Source: CAD feature listing. Evaluate the final solid. Frame: model axes, mm. A direction names the side the tool comes from. Give positions to 0.01 mm unless a question says otherwise; leave off trailing zeros. Order: outer loops, then holes, each group sorted by start corner. A loop starts at its lowest first (then second) coordinate and runs counter-clockwise, first axis right, second up.
1) Section A-A, the plane x = 0. Return loops of the section in (y, z), plus the area to 3 significant figures.
2) First-contact query: P1, Ø3.5, axis at x = -3, y = 3.5, coming from the -Z side; P2, Ø1, axis at y = 3, z = 2.5, coming from the +X side; P3, Ø3.5, axis at x = -4.5, y = 1.5, coming from the +Z side. Flat tips, straight axial feed; report the tip coordinate or a pass-through.
3) Draft query along Y for faces 4 (the face through (3, -0.05, 1)), 5 (the face through (-3.612, -0.532, 0.802)), 6 (the face through (-4.149, 3.838, 0.042)), 7 (the face through (3, -1, 0)). Return one class per face: released by +Y, released by -Y, zero draft, split by the parting line, or undercut.
4) Access query for faces 1 (the face through (2.48, 1.49, -0.33)), 2 (the face through (2.18, 4.53, -0.29)), 3 (the face through (-5.718, 2.599, -0.042)). Directions: +Z, -Z, +X, -X, +Y, -Y. A direction counts if a zero-diameter tool reaches every point of the face in a straight line with its end or side. Return the directions, or none.
5) Section B-B, the plane z = 0. Return loops of the section in (x, y), plus the area to 3 significant figures.
6) Section C-C, the plane y = 3.5. Return loops of the section in (x, z).
7) Material intervals for line 1 (Y direction, x = -3.47, z = -0.75); line 2 (X direction, y = 0.1, z = 0); line 3 (Y direction, x = -3, z = -2), sorted ascending.
8) Section D-D, the plane x = -3.47. Return loops of the section in (y, z), plus the area to 3 significant figures.
```python
from build123d import *

# Parameters (mm, degrees)
SKETCH1_R                = 3
SKETCH1_R_2              = 2.5
BOSS_EXTRUDE1_DEPTH      = 5
BOSS_EXTRUDE1_DEPTH_BACK = 1
SKETCH2_R                = 2.25
SKETCH2_R_2              = 1.5
BOSS_EXTRUDE2_DEPTH      = 3
BOSS_EXTRUDE2_DEPTH_BACK = 3
SKETCH3_R                = 1.5
CUT_EXTRUDE1_DEPTH       = 10.680826584
SKETCH4_R                = 2.5
CUT_EXTRUDE2_DEPTH       = 9.815804089
SKETCH5_R                = 0.566074209
SKETCH5_R_2              = 0.324906468
BOSS_EXTRUDE3_DEPTH      = 0.5
BOSS_EXTRUDE3_DEPTH_BACK = 0.5
SKETCH6_R                = 3.7
SKETCH6_R_2              = 3
BOSS_EXTRUDE4_DEPTH      = 0.95
SKETCH7_R                = 2.5
SKETCH7_R_2              = 2.2
BOSS_EXTRUDE5_DEPTH      = 0.95


with BuildPart() as part:
    # Sketch1 → Boss-Extrude1 (new, two sides)
    with BuildSketch(Plane(origin=(0, 0, 0), x_dir=(1, 0, 0), z_dir=(0, 1, 0))) as boss_extrude1_sk:
        with Locations(Location((0, 0, 0), (0, 0, 270))):
            Circle(SKETCH1_R)
        with Locations(Location((0, 0, 0), (0, 0, 270))):
            Circle(SKETCH1_R_2, mode=Mode.SUBTRACT)
    extrude(amount=BOSS_EXTRUDE1_DEPTH)
    extrude(boss_extrude1_sk.sketch, amount=-BOSS_EXTRUDE1_DEPTH_BACK)

    # Sketch2 → Boss-Extrude2 (add, two sides)
    with BuildSketch(Plane.XY) as boss_extrude2_sk:
        with Locations((-3.47, 2.5)):
            Circle(SKETCH2_R)
        with Locations((-3.47, 2.5)):
            Circle(SKETCH2_R_2, mode=Mode.SUBTRACT)
    extrude(amount=BOSS_EXTRUDE2_DEPTH)
    extrude(boss_extrude2_sk.sketch, amount=-BOSS_EXTRUDE2_DEPTH_BACK)

    # Sketch3 → Cut-Extrude1 (cut, through all)
    with BuildSketch(Plane.XY.offset(3)):
        with Locations((-3.47, 2.5)):
            Circle(SKETCH3_R)
    extrude(amount=-CUT_EXTRUDE1_DEPTH, mode=Mode.SUBTRACT)

    # Sketch4 → Cut-Extrude2 (cut, through all)
    with BuildSketch(Plane(origin=(0, 5, 0), x_dir=(1, 0, 0), z_dir=(0, 1, 0))):
        with Locations(Location((0, 0, 0), (0, 0, 270))):
            Circle(SKETCH4_R)
    extrude(amount=-CUT_EXTRUDE2_DEPTH, mode=Mode.SUBTRACT)

    # Sketch5 → Boss-Extrude3 (add, two sides)
    with BuildSketch(Plane.XY) as boss_extrude3_sk:
        with Locations((-3.318977868, 5.08019985)):
            Circle(SKETCH5_R)
        with Locations((-3.318977868, 5.08019985)):
            Circle(SKETCH5_R_2, mode=Mode.SUBTRACT)
    extrude(amount=BOSS_EXTRUDE3_DEPTH)
    extrude(boss_extrude3_sk.sketch, amount=-BOSS_EXTRUDE3_DEPTH_BACK)

    # Sketch6 → Boss-Extrude4 (add)
    with BuildSketch(Plane.XZ.offset(1)):
        with Locations(Location((0, 0, 0), (0, 0, 270))):
            Circle(SKETCH6_R)
        with Locations(Location((0, 0, 0), (0, 0, 170.405931773))):
            Circle(SKETCH6_R_2, mode=Mode.SUBTRACT)
    extrude(amount=-BOSS_EXTRUDE4_DEPTH)

    # Sketch7 → Boss-Extrude5 (add)
    with BuildSketch(Plane(origin=(0, 5, 0), x_dir=(1, 0, 0), z_dir=(0, 1, 0))):
        with Locations(Location((0, 0, 0), (0, 0, 270))):
            Circle(SKETCH7_R)
        with Locations(Location((0, 0, 0), (0, 0, 270))):
            Circle(SKETCH7_R_2, mode=Mode.SUBTRACT)
    extrude(amount=-BOSS_EXTRUDE5_DEPTH)


solid = part.part
```
From the geometry:
1. outline: (-1, -3.7) - (-0.05, -3.7) - (-0.05, -3) - (5, -3) - (5, -2.2) - (4.05, -2.2) - (4.05, -2.5) - (-1, -2.5) - close; (-1, 2.5) - (4.05, 2.5) - (4.05, 2.2) - (5, 2.2) - (5, 3) - (-0.05, 3) - (-0.05, 3.7) - (-1, 3.7) - close
1. area: 7.90 mm2
2. P1: stops at z = -3
2. P2: stops at x = 2.24
2. P3: stops at z = 3
3. face 4: undercut
3. face 5: zero draft
3. face 6: undercut
3. face 7: released by -Y
4. face 1: -Y
4. face 2: +Y, -Y
4. face 3: none
5. outline: (-3.76, 4.73) arc R2.25 ccw (long way) to (-3, 0.3) - (-3, -0.05) - (-3.7, -0.05) - (-3.7, -1) - (-2.5, -1) - (-2.5, 1.36) arc R1.5 cw (long way) to (-2.5, 3.64) - (-2.5, 4.05) - (-2.2, 4.05) - (-2.2, 5) - (-2.76, 5) arc R0.57 ccw (long way) to start; (2.2, 4.05) - (2.5, 4.05) - (2.5, -1) - (3.7, -1) - (3.7, -0.05) - (3, -0.05) - (3, 5) - (2.2, 5) - close; hole circle Ø0.65 at (-3.32, 5.08)
5. area: 12.2 mm2
6. outline: (-5.49, -3) - (-4.59, -3) - (-4.59, 3) - (-5.49, 3) - close; (-2.35, -3) - (-1.45, -3) - (-1.45, -2.62) arc R3 ccw (long way) to (-1.45, 2.62) - (-1.45, 3) - (-2.35, 3) - (-2.35, 0.85) arc R2.5 cw (long way) to (-2.35, -0.85) - close
7. line 1: y = -1 to -0.05, 0.25 to 1, 4 to 4.75
7. line 2: x = -3 to -2.5, 2.5 to 3
7. line 3: y = -1 to -0.05, 0.3 to 1.08, 3.92 to 4.7
8. outline: (-1, -1.28) - (-0.05, -1.28) - (-0.05, 1.28) - (-1, 1.28) - close; (0.25, -3) - (1, -3) - (1, 3) - (0.25, 3) - close; (4, -3) - (4.75, -3) - (4.75, -0.5) - (4.79, -0.5) - (4.79, 0.5) - (4.75, 0.5) - (4.75, 3) - (4, 3) - close; (5.37, -0.5) - (5.63, -0.5) - (5.63, 0.5) - (5.37, 0.5) - close
8. area: 11.7 mm2
